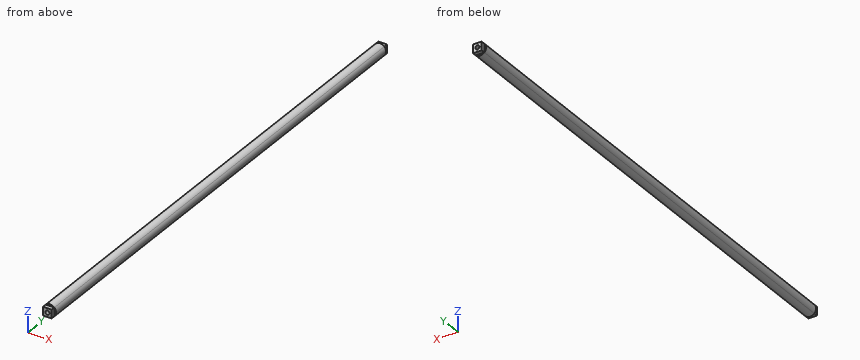
from build123d import *

# Parameters (mm, degrees)
F0_W     = 21.213204
F0_H     = 21.213204
F0_R     = 5
F1_DEPTH = 625
F2_DEPTH = 615
F3_DEPTH = 550


with BuildPart() as f1:
    # F0 (on Front) → F1 (new body, symmetric)
    with BuildSketch(Plane.XZ):
        Rectangle(F0_W, F0_H)
        Circle(F0_R, mode=Mode.SUBTRACT)
    extrude(amount=F1_DEPTH, both=True)

    # F0 (on Front) → F2 (join, symmetric)
    with BuildSketch(Plane.XZ):
        with BuildLine():
            Line((-10.606602, 10.606602), (10.606602, 10.606602))
            ThreePointArc((10.606602, 10.606602), (0, 15), (-10.606602, 10.606602))
        make_face()
        with BuildLine():
            ThreePointArc((10.606602, -10.606602), (13.858193, -5.740251), (15, 0))
            ThreePointArc((15, 0), (13.858193, 5.740251), (10.606602, 10.606602))
            Line((10.606602, 10.606602), (10.606602, -10.606602))
        make_face()
        with BuildLine():
            ThreePointArc((-10.606602, -10.606602), (0, -15), (10.606602, -10.606602))
            Line((10.606602, -10.606602), (-10.606602, -10.606602))
        make_face()
        with BuildLine():
            Line((-10.606602, -10.606602), (-10.606602, 10.606602))
            ThreePointArc((-10.606602, 10.606602), (-15, 0), (-10.606602, -10.606602))
        make_face()
    extrude(amount=F2_DEPTH, both=True)

    # F0 (on Front) → F3 (join, symmetric)
    with BuildSketch(Plane.XZ):
        Circle(F0_R)
    extrude(amount=F3_DEPTH, both=True)


solid = f1.part
Design review of the part built by this model. Coordinates are the model's own, in mm. Give positions to 0.01 mm unless a question says otherwise; leave off trailing zeros. Loops run counter-clockwise (first coordinate to the right, second up) from the corner with the lowest first, then second, coordinate; pieces in that order, holes last. Notation, with made-up numbers: M -2.5,86.5 L 42.5,86.5 A21 ccw 42.5,106.5 Z; hole C 79,38 d1. An arc over 180 degrees is marked long. Answer as a JSON object with one key per item and string values.
Item 1: For P1, Ø3, axis at y = -621, z = -0.5, coming from the +X side; P2, Ø1, axis at x = -3.5, z = 11.5, coming from the +Y side; P3, Ø9, axis at x = 0, z = 0, coming from the +Y side, all flat-tipped, find the tip position at first contact; note any pin that passes through.
Output values:
{"P1": "stops at x = 10.61", "P2": "stops at y = 615", "P3": "stops at y = 550"}
Item 2: We need section A-A (x = 0). State the section outline as (y, z) points, and give its area (3 significant figures).
Output values:
{"outline": "M -625,-10.61 L -615,-10.61 L -615,-15 L 615,-15 L 615,-10.61 L 625,-10.61 L 625,-5 L 550,-5 L 550,5 L 625,5 L 625,10.61 L 615,10.61 L 615,15 L -615,15 L -615,10.61 L -625,10.61 L -625,5 L -550,5 L -550,-5 L -625,-5 Z", "area": "35,800 mm2"}
Item 3: Wall thickness on line 1 along Z through (x, y) = (0, -575); line 2 along Z through (x, y) = (0, -342); line 3 along Z through (x, y) = (-10.5, -516.5): over which ranges is each line inside the solid? List them lowest first.
Output values:
{"line 1": "z = -15 to -5, 5 to 15", "line 2": "z = -15 to 15", "line 3": "z = -10.71 to 10.71"}
Item 4: We need section B-B (y = -475). State the section outline as (x, z) points, and give its area (3 significant figures).
Output values:
{"outline": "M -10.61,-10.61 A15 ccw 10.61,-10.61 A15 ccw 15,0 A15 ccw 10.61,10.61 A15 ccw -10.61,10.61 A15 ccw Z", "area": "707 mm2"}
